Read the model definition and answer for the solid it produces. Units are mm, in the model's axes. A direction names the side the tool comes from. Coordinates: 2 decimals unless noted, no trailing zeros. Order: outer loops, then holes, each group sorted by start corner. A loop starts at its lowest first (then second) coordinate and runs counter-clockwise, first axis right, second up. Notation, with made-up numbers: (-24.5, 29) -> (15.5, 29) arc R24 ccw to (15.5, 51) -> close; hole circle Ø10 at (-5.75, 44.5). An arc over 180 degrees is marked (long way). Return JSON: item names as keys, results as strings. Group by question number.
```python
from build123d import *

# Parameters (mm, degrees)
CROQUIS1_W              = 640
CROQUIS1_H              = 220
CROQUIS1_W_2            = 200
CROQUIS1_H_2            = 200
SALIENTE_EXTRUIR1_DEPTH = 150
CROQUIS3_W              = 640
CROQUIS3_H              = 220
SALIENTE_EXTRUIR3_DEPTH = 10
CROQUIS4_R              = 4.626495545
CORTAR_EXTRUIR1_DEPTH   = 371.135110466
CROQUIS5_W              = 640
CROQUIS5_H              = 10
CORTAR_EXTRUIR2_DEPTH   = 375.299345444
CROQUIS6_W              = 640
CROQUIS6_H              = 210
SALIENTE_EXTRUIR4_DEPTH = 20


with BuildPart() as part:
    # Croquis1 → Saliente-Extruir1 (new body)
    with BuildSketch(Plane(origin=(0, 0, 0), x_dir=(1, 0, 0), z_dir=(0, 1, 0))):
        Rectangle(CROQUIS1_W, CROQUIS1_H)
        with Locations((-210, 0)):
            Rectangle(CROQUIS1_W_2, CROQUIS1_H_2, mode=Mode.SUBTRACT)
        Rectangle(CROQUIS1_W_2, CROQUIS1_H_2, mode=Mode.SUBTRACT)
        with Locations((210, 0)):
            Rectangle(CROQUIS1_W_2, CROQUIS1_H_2, mode=Mode.SUBTRACT)
    extrude(amount=SALIENTE_EXTRUIR1_DEPTH)

    # Croquis3 → Saliente-Extruir3 (add)
    with BuildSketch(Plane.XZ):
        Rectangle(CROQUIS3_W, CROQUIS3_H)
    extrude(amount=SALIENTE_EXTRUIR3_DEPTH)

    # Croquis4 → Cortar-Extruir1 (cut, through all)
    with BuildSketch(Plane(origin=(0, 0, 0), x_dir=(1, 0, 0), z_dir=(0, 1, 0))):
        with Locations(Location((-210, 73.450625609, 0), (0, 0, 270))):
            Circle(CROQUIS4_R)
        with Locations(Location((210, 73.450625609, 0), (0, 0, 270))):
            Circle(CROQUIS4_R)
    extrude(amount=-CORTAR_EXTRUIR1_DEPTH, mode=Mode.SUBTRACT)

    # Croquis5 → Cortar-Extruir2 (cut, through all)
    with BuildSketch(Plane(origin=(0, 150, 0), x_dir=(1, 0, 0), z_dir=(0, 1, 0))):
        with Locations((0, 105)):
            Rectangle(CROQUIS5_W, CROQUIS5_H)
    extrude(amount=-CORTAR_EXTRUIR2_DEPTH, mode=Mode.SUBTRACT)

    # Croquis6 → Saliente-Extruir4 (add)
    with BuildSketch(Plane.XZ.offset(10)):
        with Locations((0, 5)):
            Rectangle(CROQUIS6_W, CROQUIS6_H)
    extrude(amount=SALIENTE_EXTRUIR4_DEPTH)


solid = part.part
```
1. Which of the six approach directions +Z, -Z, +X, -X, +Y, -Y give full straight-line access (tool end or side, diameter ignored) to faces 1 (the face through (-1, 150, 106)), 2 (the face through (-100, 74, 1))?
2. Straight lines are drawn through the part: L1, parallel to X at y = 89.5, z = -79; L2, parallel to Y at x = -146, z = -42; L3, parallel to Z at x = -13.5, y = 65. For each, find the intervals that lie inside material, in ascending order.
3. For a pull along X with two mould halves and no side action, classify faces 3 (the face through (209, 0, 1)), 4 (the face through (-211, 0, 1)), 5 (the face through (-320, 61, 4)), 6 (the face through (-4, -30, 6)) as released by +X, released by -X, zero draft, split by the parting line, or undercut.
4. Find section B-B on z = 24.5. Determine the outline of the cut face in (x, y).
5. Find section C-C on x = 72. Determine the outline of the cut face in (y, z), and give its area (3 significant figures).
6. Given pin 1 (1.5 mm diameter, centred on x = 138.5, y = 70.5, fed in from -Z); pin 2 (7.5 mm diameter, centred on x = -212, z = -72, fed in from +Y); pin 3 (8.5 mm diameter, centred on x = -210, z = -73.45, fed in from +Y), each flat-ended and moving along its own axis, determine where each tip first touches the part or whether it passes through.
7. Find section A-A on y = 80. Determine the outline of the cut face in (x, z), and give its area (3 significant figures).
Result:
{
 "1": {"face 1": "+Z, -Z, +X, -X, +Y", "face 2": "-Z, +Y"},
 "2": {"L1": "-320 to -310, -110 to -100, 100 to 110, 310 to 320", "L2": "-30 to 0", "L3": "100 to 110"},
 "3": {"face 3": "undercut", "face 4": "undercut", "face 5": "released by -X", "face 6": "zero draft"},
 "4": {"outline": "(-320, -30) -> (320, -30) -> (320, 150) -> (310, 150) -> (310, 0) -> (110, 0) -> (110, 150) -> (100, 150) -> (100, 0) -> (-100, 0) -> (-100, 150) -> (-110, 150) -> (-110, 0) -> (-310, 0) -> (-310, 150) -> (-320, 150) -> close"},
 "5": {"outline": "(-30, -100) -> (0, -100) -> (0, 100) -> (150, 100) -> (150, 110) -> (-30, 110) -> close", "area": "7,800 mm^2"},
 "6": {"pin 1": "z = 100", "pin 2": "y = 0", "pin 3": "y = -10"},
 "7": {"outline": "(-320, -100) -> (-310, -100) -> (-310, 100) -> (-110, 100) -> (-110, -100) -> (-100, -100) -> (-100, 100) -> (100, 100) -> (100, -100) -> (110, -100) -> (110, 100) -> (310, 100) -> (310, -100) -> (320, -100) -> (320, 110) -> (-320, 110) -> close", "area": "14,400 mm^2"}
}
